Geometry: see drawing. Coordinates: mm, zero at the bounding-box minimum. Coordinates: 2 decimals unless noted, no trailing zeros. Order: outer loops, then holes, each group sorted by start corner. A loop starts at its lowest first (then second) coordinate and runs counter-clockwise, first axis right, second up.
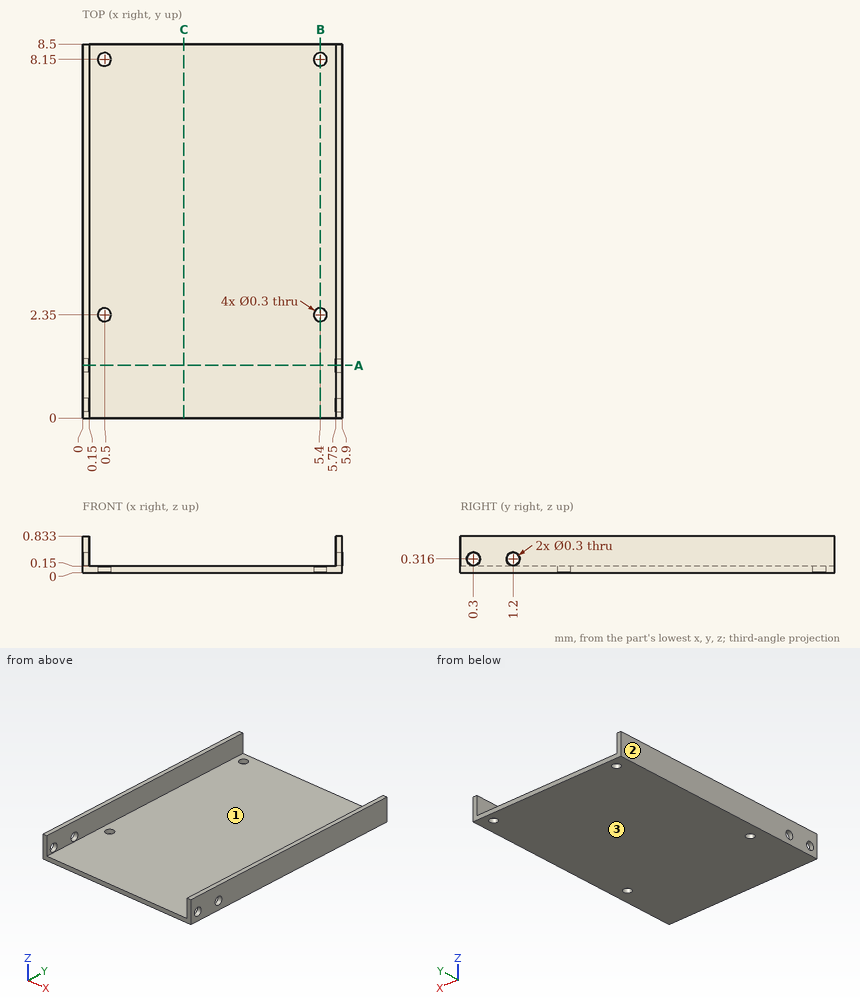
Q1. Pull-direction query (X, two-part tool) for the marked faces 1, 2 and 3; classes: pulls with the +X half, pulls with the -X half, needs draft (parallel to the pull), parting line crosses it, or undercut.
Solutions:
face 1: undercut
face 2: pulls with the -X half
face 3: needs draft
Q2. Section query A-A on y = 1.2. Give the number of separate pieces and of enclosed holes in the cut face.
Solutions:
separate pieces: 3
enclosed holes: 0
Q3. Section query C-C on x = 2.3. Output: boundary loops of the cut face in (y, z).
Solutions:
outline: (0, 0) - (8.5, 0) - (8.5, 0.15) - (0, 0.15) - close
Q4. Material intervals for line 1 along Y through (x, z) = (5.4, 0.1); line 2 along X through (y, z) = (7, 0.2); line 3 along Z through (x, y) = (4.5, 7), sorted ascending.
Solutions:
line 1: y = 0 to 2.2, 2.5 to 8, 8.3 to 8.5
line 2: x = 0 to 0.15, 5.75 to 5.9
line 3: z = 0 to 0.15
Q5. Pin query (flat end, axial travel): P1, Ø3, axis at x = 5, y = 1.5, coming from the -Z side; P2, Ø3, axis at x = 3, y = 5, coming from the +Z side. Return the tip coordinate at first contact, or that it passes through.
Solutions:
P1: stops at z = 0
P2: stops at z = 0.15
Q6. Section query B-B on x = 5.4. Output: boundary loops of the cut face in (y, z).
Solutions:
outline: (0, 0) - (2.2, 0) - (2.2, 0.15) - (0, 0.15) - close; (2.5, 0) - (8, 0) - (8, 0.15) - (2.5, 0.15) - close; (8.3, 0) - (8.5, 0) - (8.5, 0.15) - (8.3, 0.15) - close
